Geometry check sheet. Reference: drawing and pictorial views, mm from the part's lowest x, y, z. A direction names the side the tool comes from. Give positions to 0.01 mm unless a question says otherwise; leave off trailing zeros. Order: outer loops, then holes, each group sorted by start corner. A loop starts at its lowest first (then second) coordinate and runs counter-clockwise, first axis right, second up.
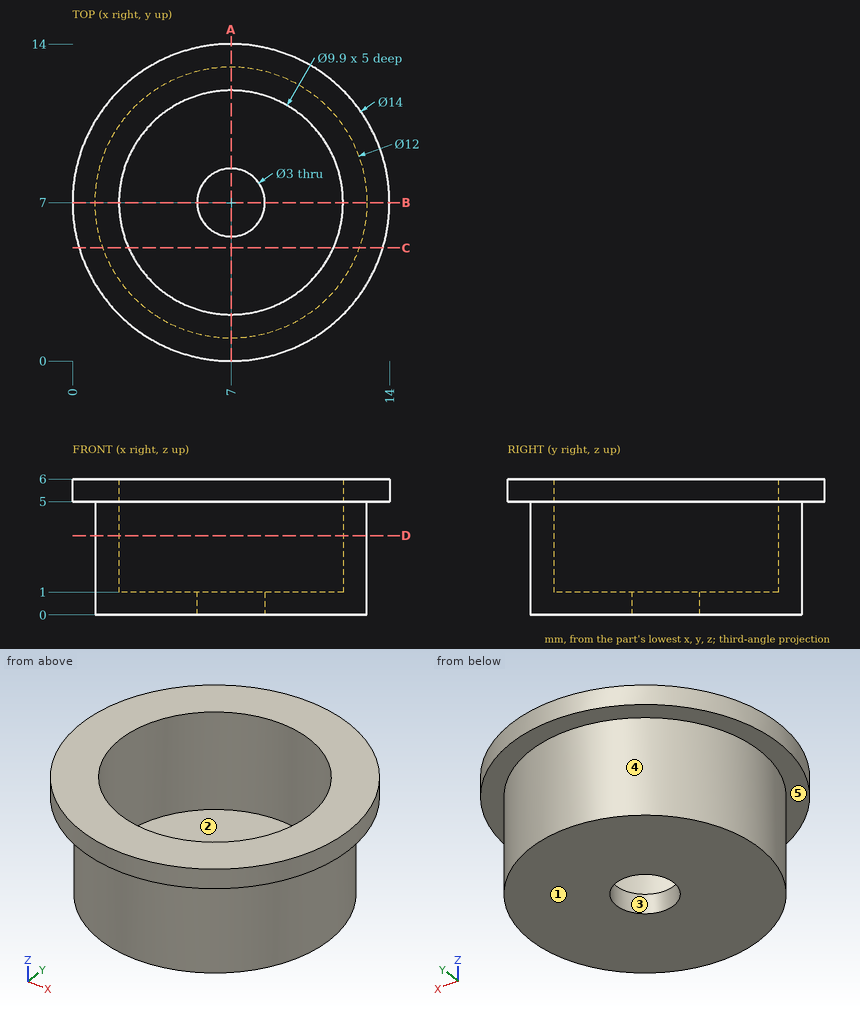
(1) Material ranges on L1, parallel to Y at x = 7, z = 2.4; L2, parallel to Y at x = 7, z = 0.6; L3, parallel to Z at x = 9.5, y = 4.5, recorded low to high.
Response values:
L1: y = 1 to 2.05, 11.95 to 13
L2: y = 1 to 5.5, 8.5 to 13
L3: z = 0 to 1
(2) Cross-section at C-C on y = 5. Enter the section's corners in (x, z).
Response values:
outline: (0.29, 5) - (1.34, 5) - (1.34, 0) - (12.66, 0) - (12.66, 5) - (13.71, 5) - (13.71, 6) - (11.53, 6) - (11.53, 1) - (2.47, 1) - (2.47, 6) - (0.29, 6) - close
(3) Gauge pin test, flat ends, axial feed: pin 1 Ø3 at (y, z) = (2, 1) entering from +X; pin 2 Ø3 at (x, y) = (8.5, 7.5) entering from +Z; pin 3 Ø2 at (y, z) = (3.5, 3) entering from +X. Record the tip position at first contact, or that the pin passes through.
Response values:
pin 1: stops at x = 11.87
pin 2: stops at z = 1
pin 3: stops at x = 12.45
(4) Set-up check for the marked faces 1 and 2: record each of +Z, -Z, +X, -X, +Y, -Y from which the full face is reachable in a straight line by a thin tool's end or side.
Response values:
face 1: -Z, +X, -X, +Y, -Y
face 2: +Z
(5) Cross-section at D-D on z = 3.5. Enter the section's corners in (x, y), then the cut area to 3 significant figures.
Response values:
outline: circle Ø12 at (7, 7); hole circle Ø9.9 at (7, 7)
area: 36.1 mm2
(6) Release check for a two-part mould opening along Y. For the marked faces 3, 4 and 5 record: released by +Y, released by -Y, zero draft, split by the parting line, or undercut.
Response values:
face 3: undercut
face 4: split by the parting line
face 5: zero draft
(7) Cross-section at A-A on x = 7. Enter the section's corners in (y, z), then the cut area to 3 significant figures.
Response values:
outline: (0, 5) - (1, 5) - (1, 0) - (5.5, 0) - (5.5, 1) - (2.05, 1) - (2.05, 6) - (0, 6) - close; (8.5, 0) - (13, 0) - (13, 5) - (14, 5) - (14, 6) - (11.95, 6) - (11.95, 1) - (8.5, 1) - close
area: 21.5 mm2
